Input: part model. Units: mm. Frame: model coordinates. A direction names the side the tool comes from. Round coordinates to 2 decimals unless told otherwise and drop trailing zeros. Write each loop counter-clockwise with the first axis right and the second up, starting at its lowest first coordinate (ties: lowest second). Pieces come first, ordered by that corner, then holes. Notation, with made-up numbers: (52.25, 47) -> (101.25, 47) arc R9 ccw to (101.25, 54) -> close; hole circle Ø1 at (82.25, 76.5). An arc over 180 degrees is marked (long way). Use CSV: the item, a comma, the result in double quotes.
```python
from build123d import *

# Parameters (mm, degrees)
SKETCH1_W           = 32
SKETCH1_H           = 32
BOSS_EXTRUDE1_DEPTH = 11
SKETCH2_W           = 28
SKETCH2_H           = 28
CUT_EXTRUDE1_DEPTH  = 7
SKETCH3_W           = 19
SKETCH3_H           = 19
CUT_EXTRUDE2_DEPTH  = 1.5
SKETCH4_W           = 17
SKETCH4_H           = 17
BOSS_EXTRUDE2_DEPTH = 1.5
SKETCH6_R           = 1.95
BOSS_EXTRUDE3_DEPTH = 9
SKETCH7_R           = 1.5
CUT_EXTRUDE3_DEPTH  = 3


with BuildPart() as part:
    # Sketch1 → Boss-Extrude1 (new body)
    with BuildSketch(Plane(origin=(0, 0, 0), x_dir=(1, 0, 0), z_dir=(0, 1, 0))):
        Rectangle(SKETCH1_W, SKETCH1_H)
    extrude(amount=BOSS_EXTRUDE1_DEPTH)

    # Sketch2 → Cut-Extrude1 (cut)
    with BuildSketch(Plane(origin=(0, 11, 0), x_dir=(1, 0, 0), z_dir=(0, 1, 0))):
        Rectangle(SKETCH2_W, SKETCH2_H)
    extrude(amount=-CUT_EXTRUDE1_DEPTH, mode=Mode.SUBTRACT)

    # Sketch3 → Cut-Extrude2 (cut)
    with BuildSketch(Plane(origin=(0, 4, 0), x_dir=(1, 0, 0), z_dir=(0, 1, 0))):
        Rectangle(SKETCH3_W, SKETCH3_H)
    extrude(amount=-CUT_EXTRUDE2_DEPTH, mode=Mode.SUBTRACT)

    # Sketch4 → Boss-Extrude2 (add)
    with BuildSketch(Plane(origin=(0, 2.5, 0), x_dir=(1, 0, 0), z_dir=(0, 1, 0))):
        Rectangle(SKETCH4_W, SKETCH4_H)
    extrude(amount=BOSS_EXTRUDE2_DEPTH)

    # Sketch6 → Boss-Extrude3 (add)
    with BuildSketch(Plane(origin=(0, 4, 0), x_dir=(1, 0, 0), z_dir=(0, 1, 0))):
        with Locations((-11.75, 11.75)):
            Circle(SKETCH6_R)
        with Locations((11.75, 11.75)):
            Circle(SKETCH6_R)
        with Locations((11.75, -11.75)):
            Circle(SKETCH6_R)
        with Locations((-11.75, -11.75)):
            Circle(SKETCH6_R)
    extrude(amount=BOSS_EXTRUDE3_DEPTH)

    # Sketch7 → Cut-Extrude3 (cut)
    with BuildSketch(Plane(origin=(0, 4, 0), x_dir=(1, 0, 0), z_dir=(0, 1, 0))):
        with Locations((-6, -6)):
            Circle(SKETCH7_R)
        with Locations((-2, -6)):
            Circle(SKETCH7_R)
        with Locations((2, -6)):
            Circle(SKETCH7_R)
        with Locations((6, -6)):
            Circle(SKETCH7_R)
        with Locations((-2, -2)):
            Circle(SKETCH7_R)
        with Locations((2, -2)):
            Circle(SKETCH7_R)
        with Locations((6, -2)):
            Circle(SKETCH7_R)
        with Locations((-2, 2)):
            Circle(SKETCH7_R)
        with Locations((2, 2)):
            Circle(SKETCH7_R)
        with Locations((6, 2)):
            Circle(SKETCH7_R)
        with Locations((-2, 6)):
            Circle(SKETCH7_R)
        with Locations((2, 6)):
            Circle(SKETCH7_R)
        with Locations((6, 6)):
            Circle(SKETCH7_R)
        with Locations((-6, -2)):
            Circle(SKETCH7_R)
        with Locations((-6, 2)):
            Circle(SKETCH7_R)
        with Locations((-6, 6)):
            Circle(SKETCH7_R)
    extrude(amount=-CUT_EXTRUDE3_DEPTH, mode=Mode.SUBTRACT)


solid = part.part
```
Item 1: Set-up query: faces 4 (the face through (-12, 13, -12)), 5 (the face through (2, 1, -2)). Return all of +Z, -Z, +X, -X, +Y, -Y with unobstructed straight access to the full face (end or side cutting, diameter ignored); none if empty.
Worked answers:
face 4,"+Z, -Z, +X, -X, +Y"
face 5,"+Y"
Item 2: First-contact query: pin 1 Ø3.5 at (x, z) = (2, 6) entering from +Y; pin 2 Ø1.5 at (x, z) = (-5.5, -6) entering from +Y. Flat tips, straight axial feed; report the tip coordinate or a pass-through.
Worked answers:
pin 1,"stops at y = 4"
pin 2,"stops at y = 1"
Item 3: Line query: line 1 (Z direction, x = -2, y = 1.75); line 2 (X direction, y = 4.25, z = 6.5). Output: solid intervals per line, ascending.
Worked answers:
line 1,"z = -16 to -7.5, -4.5 to -3.5, -0.5 to 0.5, 3.5 to 4.5, 7.5 to 16"
line 2,"x = -16 to -14, 14 to 16"
Item 4: Pull-direction query (X, two-part tool) for faces 1 (the face through (12, 13, 12)), 2 (the face through (-16, 5, 0)), 3 (the face through (14, 8, 0)); classes: +X half, -X half, draft (parallel to the pull), parting line (faces both ways), or undercut.
Worked answers:
face 1,"draft"
face 2,"-X half"
face 3,"undercut"
Item 5: Section query A-A on y = 3. Give the number of separate pieces and of enclosed holes in the cut face, plus the area to 3 significant figures.
Worked answers:
separate pieces,"2"
enclosed holes,"17"
area,"839 mm²"
Item 6: Section query B-B on y = 5. Return the cut outline in (x, z).
Worked answers:
outline,"(-16, -16) -> (16, -16) -> (16, 16) -> (-16, 16) -> close; circle Ø3.9 at (-11.75, -11.75); circle Ø3.9 at (-11.75, 11.75); circle Ø3.9 at (11.75, -11.75); circle Ø3.9 at (11.75, 11.75); hole (-14, -14) -> (14, -14) -> (14, 14) -> (-14, 14) -> close"
Item 7: Section query D-D on z = -11.75. Return the cut outline in (x, y), plus the area to 3 significant figures.
Worked answers:
outline,"(-16, 0) -> (16, 0) -> (16, 11) -> (14, 11) -> (14, 4) -> (13.7, 4) -> (13.7, 13) -> (9.8, 13) -> (9.8, 4) -> (-9.8, 4) -> (-9.8, 13) -> (-13.7, 13) -> (-13.7, 4) -> (-14, 4) -> (-14, 11) -> (-16, 11) -> close"
area,"226 mm²"
